Here's how the part is built. I have some questions about the finished solid (model axes, mm). Face numbers are marked on the shaded views. A direction names the side the tool comes from. Round coordinates to 2 decimals unless told otherwise and drop trailing zeros. Write each loop counter-clockwise with the first axis right and the second up, starting at its lowest first coordinate (ties: lowest second). Pieces come first, ordered by that corner, then holes. Notation, with made-up numbers: (74, -30.5) -> (104, -30.5) arc R7 ccw to (104, -19.5) -> close; hole circle Ø1 at (54.25, 11). An arc over 180 degrees is marked (long way). Put each result on its own line as item: value. Start each with the question number.
1. We'd pull the mould along Z, two halves only. Please class the marked faces 1, 2, 3 and 4: +Z half, -Z half, draft (parallel to the pull), parting line (faces both ways), or undercut.
2. I need wall thicknesses on probe 1 along X at (y, z) = (6, 0); probe 2 along Y at (x, z) = (-12, -1); probe 3 along Z at (x, y) = (10.5, 4.25). Which ranges of each line are inside material? Lowest first, please. Write a range as from..to.
3. Which directions (+Z, -Z, +X, -X, +Y, -Y) give clear straight access to the entire face, cutting with the end or side of a thin tool? Please do the marked faces 5 and 6.
4. For pin 1 (19.5 mm diameter, centred on x = 4.35, z = 0, fed in from +Y); pin 2 (6 mm diameter, centred on x = -3.5, y = 8.5, fed in from +Z); pin 3 (1.5 mm diameter, centred on y = 7.5, z = -5.5, fed in from -X), each with a flat end and sliding along its axis, tell me the tip position at first contact or that it passes through.
5. Suppose I cut it at B-B (x = 4.35). Please give me the cut outline in (y, z), then the cut area to 3 significant figures.
6. Suppose I cut it at C-C (y = 6.5). Please give me the cut outline in (x, z), then the cut area to 3 significant figures.
7. Suppose I cut it at A-A (z = 14.6). Please give me the cut outline in (x, y).
8. Suppose I cut it at D-D (z = 0). Please give me the cut outline in (x, y).
```python
from build123d import *

# Parameters (mm, degrees)
SKETCH1_R           = 11.8
SKETCH1_R_2         = 1
BOSS_EXTRUDE1_DEPTH = 3
SKETCH3_R           = 11.8
BOSS_EXTRUDE2_DEPTH = 11
SHELL1_T            = -1
SKETCH4_R           = 2.5
CUT_EXTRUDE2_DEPTH  = 3
BOSS_EXTRUDE4_DEPTH = 7
SKETCH6_R           = 2.5
CUT_EXTRUDE3_DEPTH  = 27.895771043


with BuildPart() as part:
    # Sketch1 → Boss-Extrude1 (new body)
    with BuildSketch(Plane(origin=(0, 0, 0), x_dir=(1, 0, 0), z_dir=(0, 1, 0))):
        with BuildLine():
            Line((-17.15, 16.6), (17.15, 16.6))
            ThreePointArc((17.15, 16.6), (18.210660172, 16.160660172), (18.65, 15.1))
            Line((18.65, 15.1), (18.65, -15.1))
            ThreePointArc((18.65, -15.1), (18.210660172, -16.160660172), (17.15, -16.6))
            Line((17.15, -16.6), (-17.15, -16.6))
            ThreePointArc((-17.15, -16.6), (-18.210660172, -16.160660172), (-18.65, -15.1))
            Line((-18.65, -15.1), (-18.65, 15.1))
            ThreePointArc((-18.65, 15.1), (-18.210660172, 16.160660172), (-17.15, 16.6))
        make_face()
        with Locations(Location((4.35, 0, 0), (0, 0, 270))):
            Circle(SKETCH1_R, mode=Mode.SUBTRACT)
        with Locations(Location((-16.403012048, 14.6, 0), (0, 0, 270))):
            Circle(SKETCH1_R_2, mode=Mode.SUBTRACT)
        with Locations(Location((16.403012048, 14.6, 0), (0, 0, 90))):
            Circle(SKETCH1_R_2, mode=Mode.SUBTRACT)
        with Locations(Location((16.403012048, -14.6, 0), (0, 0, 270))):
            Circle(SKETCH1_R_2, mode=Mode.SUBTRACT)
        with Locations(Location((-16.403012048, -14.6, 0), (0, 0, 90))):
            Circle(SKETCH1_R_2, mode=Mode.SUBTRACT)
    extrude(amount=BOSS_EXTRUDE1_DEPTH)

    # Sketch3 → Boss-Extrude2 (add)
    with BuildSketch(Plane(origin=(0, 0, 0), x_dir=(1, 0, 0), z_dir=(0, 1, 0))):
        with Locations(Location((4.35, 0, 0), (0, 0, 270))):
            Circle(SKETCH3_R)
    extrude(amount=BOSS_EXTRUDE2_DEPTH)

    # Shell1
    shell1_openings = [part.faces().sort_by_distance(p)[0] for p in [
        (4.35, 11, 0),
    ]]
    offset(amount=SHELL1_T, openings=shell1_openings, kind=Kind.INTERSECTION)

    # Sketch4 → Cut-Extrude2 (cut)
    with BuildSketch(Plane.XZ):
        with Locations(Location((4.35, 0, 0), (0, 0, 270))):
            Circle(SKETCH4_R)
    extrude(amount=-CUT_EXTRUDE2_DEPTH, mode=Mode.SUBTRACT)

    # Sketch5 → Boss-Extrude4 (add)
    with BuildSketch(Plane(origin=(0, 1, 0), x_dir=(1, 0, 0), z_dir=(0, 1, 0))):
        with BuildLine():
            Line((2.02679539, 7.505692886), (2.465229351, 2.97646884))
            ThreePointArc((2.465229351, 2.97646884), (2.176988688, 2.173011312), (1.37353116, 1.884770649))
            Line((1.37353116, 1.884770649), (-3.155692886, 2.32320461))
            ThreePointArc((-3.155692886, 2.32320461), (-5.478897496, 0), (-3.155692886, -2.32320461))
            Line((-3.155692886, -2.32320461), (1.37353116, -1.884770649))
            ThreePointArc((1.37353116, -1.884770649), (2.176988688, -2.173011312), (2.465229351, -2.97646884))
            Line((2.465229351, -2.97646884), (2.02679539, -7.505692886))
            ThreePointArc((2.02679539, -7.505692886), (4.35, -9.828897496), (6.67320461, -7.505692886))
            Line((6.67320461, -7.505692886), (6.234770649, -2.97646884))
            ThreePointArc((6.234770649, -2.97646884), (6.523011312, -2.173011312), (7.32646884, -1.884770649))
            Line((7.32646884, -1.884770649), (11.855692886, -2.32320461))
            ThreePointArc((11.855692886, -2.32320461), (14.178897496, 0), (11.855692886, 2.32320461))
            Line((11.855692886, 2.32320461), (7.32646884, 1.884770649))
            ThreePointArc((7.32646884, 1.884770649), (6.523011312, 2.173011312), (6.234770649, 2.97646884))
            Line((6.234770649, 2.97646884), (6.67320461, 7.505692886))
            ThreePointArc((6.67320461, 7.505692886), (4.35, 9.828897496), (2.02679539, 7.505692886))
        make_face()
    extrude(amount=BOSS_EXTRUDE4_DEPTH)

    # Sketch6 → Cut-Extrude3 (cut, through all)
    with BuildSketch(Plane.XZ.offset(-1)):
        with Locations(Location((4.35, 0, 0), (0, 0, 270))):
            Circle(SKETCH6_R)
    extrude(amount=-CUT_EXTRUDE3_DEPTH, mode=Mode.SUBTRACT)


solid = part.part
```
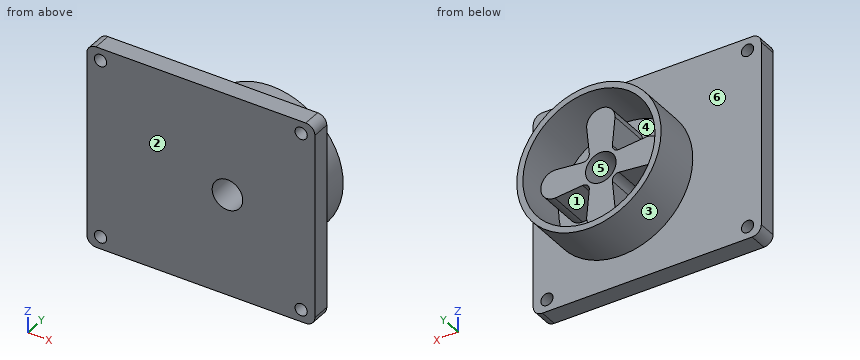
Verdict:
1. face 1: undercut
1. face 2: draft
1. face 3: parting line
1. face 4: undercut
2. probe 1: x = -7.45..-6.45, -5.48..1.85, 6.85..14.18, 15.15..16.15
2. probe 2: y = 0..1, 2..3
2. probe 3: z = -10.07..-8.88, -2.19..2.19, 8.88..10.07
3. face 5: +Y, -Y
3. face 6: +Y
4. pin 1: stops at y = 8
4. pin 2: stops at z = 10.76
4. pin 3: stops at x = -6.45
5. outline: (0, -16.6) -> (3, -16.6) -> (3, -11.8) -> (11, -11.8) -> (11, -10.8) -> (2, -10.8) -> (2, -15.6) -> (1, -15.6) -> (1, -9.83) -> (8, -9.83) -> (8, -2.5) -> (0, -2.5) -> close; (0, 2.5) -> (8, 2.5) -> (8, 9.83) -> (1, 9.83) -> (1, 15.6) -> (2, 15.6) -> (2, 10.8) -> (11, 10.8) -> (11, 11.8) -> (3, 11.8) -> (3, 16.6) -> (0, 16.6) -> close
5. area: 160 mm^2
6. outline: circle Ø23.6 at (4.35, 0); (-3.16, -2.32) -> (1.37, -1.88) arc R1 cw to (2.47, -2.98) -> (2.03, -7.51) arc R2.32 ccw to (6.67, -7.51) -> (6.23, -2.98) arc R1 cw to (7.33, -1.88) -> (11.86, -2.32) arc R2.32 ccw to (11.86, 2.32) -> (7.33, 1.88) arc R1 cw to (6.23, 2.98) -> (6.67, 7.51) arc R2.32 ccw to (2.03, 7.51) -> (2.47, 2.98) arc R1 cw to (1.37, 1.88) -> (-3.16, 2.32) arc R2.32 ccw to start; hole circle Ø21.6 at (4.35, 0); hole circle Ø5 at (4.35, 0)
6. area: 193 mm^2
7. outline: (-18.65, 0) -> (-17.4, 0) -> (-17.4, 3) -> (-18.65, 3) -> close; (-15.4, 0) -> (15.4, 0) -> (15.4, 3) -> (-15.4, 3) -> close; (17.4, 0) -> (18.65, 0) -> (18.65, 3) -> (17.4, 3) -> close; hole (-14.4, 1) -> (14.4, 1) -> (14.4, 2) -> (-14.4, 2) -> close
8. outline: (-18.65, 0) -> (1.85, 0) -> (1.85, 8) -> (-5.48, 8) -> (-5.48, 1) -> (-17.65, 1) -> (-17.65, 2) -> (-6.45, 2) -> (-6.45, 11) -> (-7.45, 11) -> (-7.45, 3) -> (-18.65, 3) -> close; (6.85, 0) -> (18.65, 0) -> (18.65, 3) -> (16.15, 3) -> (16.15, 11) -> (15.15, 11) -> (15.15, 2) -> (17.65, 2) -> (17.65, 1) -> (14.18, 1) -> (14.18, 8) -> (6.85, 8) -> close
